Verification items for the finished model (mm, model axes). A direction names the side the tool comes from. Round coordinates to 2 decimals unless told otherwise and drop trailing zeros. Write each loop counter-clockwise with the first axis right and the second up, starting at its lowest first coordinate (ties: lowest second). Pieces come first, ordered by that corner, then holes. Notation, with made-up numbers: M -2,9.5 L 43,9.5 A21 ccw 43,13.5 Z; hole C 52.25,4 d10. An arc over 180 degrees is marked long. Write each question's results on one line, items separated by ' | '.
from build123d import *
from build123d.topology import SkipClean

# Parameters (mm, degrees)
SKETCH1_W                = 50
SKETCH1_H                = 25
SKETCH1_R                = 1.3
SKETCH1_R_2              = 4.5
BOSS_EXTRUDE1_DEPTH      = 2.5
SKETCH2_W                = 50
SKETCH2_H                = 12
BOSS_EXTRUDE2_DEPTH      = 3
SKETCH3_W                = 50
SKETCH3_H                = 28
BOSS_EXTRUDE3_DEPTH      = 3
SKETCH4_R                = 1.3
CUT_EXTRUDE1_DEPTH       = 34.018933962
SKETCH5_W                = 53
SKETCH5_H                = 32.5
SKETCH5_R                = 1.6
SKETCH5_W_2              = 42
SKETCH5_H_2              = 21.5
BOSS_EXTRUDE4_DEPTH      = 4
SKETCH7_R                = 8
CUT_EXTRUDE2_DEPTH       = 5
SKETCH8_W                = 24.55
SKETCH8_H                = 21.5
CUT_EXTRUDE3_DEPTH       = 3.8
BOSS_EXTRUDE6_DEPTH      = 22.95
BOSS_EXTRUDE7_DEPTH      = 2
CUT_EXTRUDE4_START       = -1.2
SKETCH11_R               = 1.6
CUT_EXTRUDE4_DEPTH       = 1.2
SKETCH12_W               = 7
SKETCH12_H               = 21
SKETCH12_R               = 1.6
BOSS_EXTRUDE8_DEPTH      = 7.8
CUT_EXTRUDE5_DEPTH       = 55.054972019
CUT_EXTRUDE5_DEPTH_BACK  = 55.054972019
SKETCH13_W               = 0.7
SKETCH13_H               = 5
SKETCH13_H_2             = 4
CUT_EXTRUDE6_DEPTH       = 78.713850117
CUT_EXTRUDE6_DEPTH_BACK  = 78.713850117
SKETCH14_W               = 28
SKETCH14_H               = 10
SKETCH16_R               = 3
CUT_EXTRUDE8_DEPTH       = 3
SKETCH15_R               = 1.6
CUT_EXTRUDE9_DEPTH       = 5
SKETCH17_W               = 16.3
SKETCH17_H               = 5
CUT_EXTRUDE10_DEPTH      = 3.2
SKETCH18_R               = 1.45
CUT_EXTRUDE11_DEPTH      = 5
CUT_EXTRUDE12_DEPTH      = 54.307527611
CUT_EXTRUDE12_DEPTH_BACK = 54.307527611
SKETCH19_R               = 1.6
CUT_EXTRUDE14_DEPTH      = 60.569224437
CUT_EXTRUDE14_DEPTH_BACK = 60.569224437
SKETCH20_W               = 17.95
SKETCH20_H               = 5
BOSS_EXTRUDE11_START     = 2
SKETCH21_W               = 16.3
SKETCH21_H               = 5
SKETCH21_R               = 1.45
BOSS_EXTRUDE11_DEPTH     = 2


with BuildPart() as part:
    # Sketch1 → Boss-Extrude1 (new, symmetric)
    with BuildSketch(Plane(origin=(0, 0, 0), x_dir=(1, 0, 0), z_dir=(0, 1, 0))):
        Rectangle(SKETCH1_W, SKETCH1_H)
        with Locations(Location((-11.25, 0, 0), (0, 0, 270))):
            Circle(SKETCH1_R, mode=Mode.SUBTRACT)
        with Locations(Location((11.25, 0, 0), (0, 0, 270))):
            Circle(SKETCH1_R_2, mode=Mode.SUBTRACT)
    extrude(amount=BOSS_EXTRUDE1_DEPTH, both=True)

    # Sketch2 → Boss-Extrude2 (add)
    with BuildSketch(Plane.XY.offset(12.5)):
        with Locations((0, 3.5)):
            Rectangle(SKETCH2_W, SKETCH2_H)
    extrude(amount=BOSS_EXTRUDE2_DEPTH)

    # Sketch3 → Boss-Extrude3 (add)
    with BuildSketch(Plane(origin=(0, 9.5, 0), x_dir=(1, 0, 0), z_dir=(0, 1, 0))):
        with Locations((0, -1.5)):
            Rectangle(SKETCH3_W, SKETCH3_H)
    extrude(amount=BOSS_EXTRUDE3_DEPTH)

    # Sketch4 → Cut-Extrude1 (cut, through all)
    with BuildSketch(Plane(origin=(0, 12.5, 0), x_dir=(1, 0, 0), z_dir=(0, 1, 0))):
        with Locations(Location((11.25, 0, 0), (0, 0, 270))):
            Circle(SKETCH4_R)
        with Locations(Location((-11.25, 0, 0), (0, 0, 270))):
            Circle(SKETCH4_R)
    extrude(amount=-CUT_EXTRUDE1_DEPTH, mode=Mode.SUBTRACT)

    # Sketch5 → Boss-Extrude4 (add)
    with BuildSketch(Plane.XZ.offset(2.5)):
        with Locations((21.45, -0.05)):
            Rectangle(SKETCH5_W, SKETCH5_H)
        with Locations(Location((45.75, -5, 0), (0, 0, 270))):
            Circle(SKETCH5_R, mode=Mode.SUBTRACT)
        with Locations(Location((45.75, 4.9, 0), (0, 0, 270))):
            Circle(SKETCH5_R, mode=Mode.SUBTRACT)
        with Locations(Location((-2.85, 4.9, 0), (0, 0, 270))):
            Circle(SKETCH5_R, mode=Mode.SUBTRACT)
        with Locations(Location((-2.85, -5, 0), (0, 0, 270))):
            Circle(SKETCH5_R, mode=Mode.SUBTRACT)
        with Locations((21.45, -0.05)):
            Rectangle(SKETCH5_W_2, SKETCH5_H_2, mode=Mode.SUBTRACT)
    extrude(amount=BOSS_EXTRUDE4_DEPTH)

    # Sketch7 → Cut-Extrude2 (cut)
    with BuildSketch(Plane.XZ.offset(2.5)):
        with Locations(Location((11.25, 0, 0), (0, 0, 270))):
            Circle(SKETCH7_R)
    extrude(amount=-CUT_EXTRUDE2_DEPTH, mode=Mode.SUBTRACT)

    # Sketch8 → Cut-Extrude3 (cut)
    with BuildSketch(Plane.XZ.offset(2.5)):
        with Locations((12.725, -0.05)):
            Rectangle(SKETCH8_W, SKETCH8_H)
    extrude(amount=-CUT_EXTRUDE3_DEPTH, mode=Mode.SUBTRACT)

    # Sketch9 → Boss-Extrude6 (add)
    with BuildSketch(Plane(origin=(25, 0, 0), x_dir=(0, 0, -1), z_dir=(1, 0, 0))):
        Polygon((12.5, 2.5), (-16.2, 2.5), (-16.2, -2.5), (-10.7, -2.5), (-10.7, 1.3), (10.8, 1.3), (10.8, -2.5), (12.5, -2.5), align=None)
    extrude(amount=BOSS_EXTRUDE6_DEPTH)

    # Sketch10 → Boss-Extrude7 (add)
    with BuildSketch(Plane(origin=(47.95, 0, 0), x_dir=(0, 0, -1), z_dir=(1, 0, 0))):
        Polygon((16.3, -2.5), (12.5, -2.5), (12.5, 2.5), (-16.2, 2.5), (-16.2, -6.5), (16.3, -6.5), align=None)
    extrude(amount=BOSS_EXTRUDE7_DEPTH)

    # Sketch11 → Cut-Extrude4 (cut)
    with BuildSketch(Plane.XZ.offset(-1.3).offset(CUT_EXTRUDE4_START)):
        with Locations(Location((-2.85, 4.9, 0), (0, 0, 270))):
            Circle(SKETCH11_R)
        with Locations(Location((-2.85, -5, 0), (0, 0, 270))):
            Circle(SKETCH11_R)
        with Locations(Location((45.75, 4.9, 0), (0, 0, 270))):
            Circle(SKETCH11_R)
        with Locations(Location((45.75, -5, 0), (0, 0, 270))):
            Circle(SKETCH11_R)
    extrude(amount=CUT_EXTRUDE4_DEPTH, mode=Mode.SUBTRACT)

    # Sketch12 → Boss-Extrude8 (add)
    with BuildSketch(Plane.XZ.offset(-1.3)):
        with Locations((46.45, 0.2)):
            Rectangle(SKETCH12_W, SKETCH12_H)
        with Locations(Location((45.75, 4.9, 0), (0, 0, 90))):
            Circle(SKETCH12_R, mode=Mode.SUBTRACT)
        with Locations(Location((45.75, -5, 0), (0, 0, 90))):
            Circle(SKETCH12_R, mode=Mode.SUBTRACT)
    extrude(amount=BOSS_EXTRUDE8_DEPTH)

    # Sketch13 → Cut-Extrude5 (cut, two sides: drawn at the far end of the back side and taken through both)
    with BuildSketch(Plane.ZY.offset(-25).offset(-CUT_EXTRUDE5_DEPTH_BACK)):
        with Locations((15.85, 0)):
            Rectangle(SKETCH13_W, SKETCH13_H)
        with Locations((15.85, -4.5)):
            Rectangle(SKETCH13_W, SKETCH13_H_2)
    extrude(amount=CUT_EXTRUDE5_DEPTH + CUT_EXTRUDE5_DEPTH_BACK, mode=Mode.SUBTRACT)

    # Sketch14 → Cut-Extrude6 (cut, two sides: drawn at the far end of the back side and taken through both)
    with BuildSketch(Plane.ZY.offset(25).offset(-CUT_EXTRUDE6_DEPTH_BACK)):
        with Locations((1.5, 7.5)):
            Rectangle(SKETCH14_W, SKETCH14_H)
    extrude(amount=CUT_EXTRUDE6_DEPTH + CUT_EXTRUDE6_DEPTH_BACK, mode=Mode.SUBTRACT)

    # Sketch16 → Cut-Extrude8 (cut)
    with BuildSketch(Plane(origin=(0, 2.5, 0), x_dir=(1, 0, 0), z_dir=(0, 1, 0))):
        with Locations(Location((-2.85, 5, 0), (0, 0, 270))):
            Circle(SKETCH16_R)
        with Locations(Location((-2.85, -4.9, 0), (0, 0, 270))):
            Circle(SKETCH16_R)
        with Locations(Location((45.75, 5, 0), (0, 0, 270))):
            Circle(SKETCH16_R)
        with Locations(Location((45.75, -4.9, 0), (0, 0, 270))):
            Circle(SKETCH16_R)
    extrude(amount=-CUT_EXTRUDE8_DEPTH, mode=Mode.SUBTRACT)

    # Sketch15 → Cut-Extrude9 (cut)
    with SkipClean():  # the faces are left unmerged after this step: merging them gives an invalid solid
        with BuildSketch(Plane(origin=(0, 2.5, 0), x_dir=(1, 0, 0), z_dir=(0, 1, 0))):
            with Locations(Location((-2.85, 5, 0), (0, 0, 270))):
                Circle(SKETCH15_R)
            with Locations(Location((-2.85, -4.9, 0), (0, 0, 270))):
                Circle(SKETCH15_R)
        extrude(amount=-CUT_EXTRUDE9_DEPTH, mode=Mode.SUBTRACT)

    # Sketch17 → Cut-Extrude10 (cut)
    with SkipClean():  # the faces are left unmerged after this step: merging them gives an invalid solid
        with BuildSketch(Plane.XY.offset(15.5)):
            with Locations((8.9, 0)):
                Rectangle(SKETCH17_W, SKETCH17_H)
            with Locations((31, 0)):
                Rectangle(SKETCH17_W, SKETCH17_H)
        extrude(amount=-CUT_EXTRUDE10_DEPTH, mode=Mode.SUBTRACT)

    # Sketch18 → Cut-Extrude11 (cut)
    with SkipClean():  # the faces are left unmerged after this step: merging them gives an invalid solid
        with BuildSketch(Plane.XY.offset(12.3)):
            with Locations((8.95, 0)):
                Circle(SKETCH18_R)
            with Locations((30.95, 0)):
                Circle(SKETCH18_R)
        extrude(amount=-CUT_EXTRUDE11_DEPTH, mode=Mode.SUBTRACT)

    # Sketch19 → Cut-Extrude12 (cut, two sides: drawn at the far end of the back side and taken through both)
    with SkipClean():  # the faces are left unmerged after this step: merging them gives an invalid solid
        with BuildSketch(Plane(origin=(0, 2.5, 0), x_dir=(1, 0, 0), z_dir=(0, 1, 0)).offset(-CUT_EXTRUDE12_DEPTH_BACK)):
            with Locations(Location((33.75, 0, 0), (0, 0, 270))):
                Circle(SKETCH19_R)
        extrude(amount=CUT_EXTRUDE12_DEPTH + CUT_EXTRUDE12_DEPTH_BACK, mode=Mode.SUBTRACT)

    # Sketch20 → Cut-Extrude14 (cut, two sides: drawn at the far end of the back side and taken through both)
    with SkipClean():  # the faces are left unmerged after this step: merging them gives an invalid solid
        with BuildSketch(Plane.XY.offset(15.5).offset(-CUT_EXTRUDE14_DEPTH_BACK)):
            with Locations((-16.025, 0)):
                Rectangle(SKETCH20_W, SKETCH20_H)
        extrude(amount=CUT_EXTRUDE14_DEPTH + CUT_EXTRUDE14_DEPTH_BACK, mode=Mode.SUBTRACT)

    # Sketch21 → Boss-Extrude11 (add)
    # profile 1 of 3: a face of its own
    with SkipClean():  # the faces are left unmerged after this step: merging them gives an invalid solid
        with BuildSketch(Plane.XY.offset(15.5).offset(BOSS_EXTRUDE11_START)):
            with Locations((8.9, 0)):
                Rectangle(SKETCH21_W, SKETCH21_H)
            with Locations((8.95, 0)):
                Circle(SKETCH21_R, mode=Mode.SUBTRACT)
        # profile 2 of 3: a face of its own
        with BuildSketch(Plane.XY.offset(15.5).offset(BOSS_EXTRUDE11_START)):
            Polygon((0.75, -2.5), (0.75, 2.5), (-7.05, 2.5), (-7.05, -2.5), (-5.05, -2.5), (-5.05, -6.5), (49.95, -6.5), (49.95, 2.5), (39.15, 2.5), (39.15, -2.5), (22.85, -2.5), (22.85, 2.5), (17.05, 2.5), (17.05, -2.5), align=None)
        # profile 3 of 3: a face of its own
        with BuildSketch(Plane.XY.offset(15.5).offset(BOSS_EXTRUDE11_START)):
            with Locations((31, 0)):
                Rectangle(SKETCH21_W, SKETCH21_H)
            with Locations((30.95, 0)):
                Circle(SKETCH21_R, mode=Mode.SUBTRACT)
        extrude(amount=-BOSS_EXTRUDE11_DEPTH)


solid = part.part
1) Sectioned sample at D-D, the plane z = -5. Count the separate pieces of the cut face and the enclosed holes in it, and give its area (3 significant figures).
Calculated:
separate pieces: 5 | enclosed holes: 0 | area: 86.5 mm²
2) Sectioned sample at B-B, the plane x = 11.25. Record the cut outline in (y, z).
Calculated:
outline: M -6.5,-16.3 L -2.5,-16.3 L -2.5,-12.5 L 2.5,-12.5 L 2.5,-8 L 1.3,-8 L 1.3,-10.8 L -6.5,-10.8 Z; M -6.5,10.7 L 1.3,10.7 L 1.3,8 L 2.5,8 L 2.5,12.3 L -2.5,12.3 L -2.5,15.5 L 2.5,15.5 L 2.5,17.5 L -6.5,17.5 Z
3) Sectioned sample at A-A, the plane z = 0. Record the cut outline in (x, y).
Calculated:
outline: M -7.05,-2.5 L -5.05,-2.5 L -5.05,-6.5 L 0.45,-6.5 L 0.45,1.3 L 3.25,1.3 L 3.25,2.5 L -7.05,2.5 Z; M 19.25,1.3 L 32.15,1.3 L 32.15,2.5 L 19.25,2.5 Z; M 35.35,1.3 L 42.95,1.3 L 42.95,-2.5 L 42.45,-2.5 L 42.45,-6.5 L 49.95,-6.5 L 49.95,2.5 L 35.35,2.5 Z
4) Draft check along X on faces 5 (the flat face through (0.45, -3, 0)), 6 (the flat face through (21, -2, 17.5)), 7 (the flat face through (-4.1, -0.5, 6.2)), 8 (the flat face through (-5.05, -4, 1)). Enter one of: pulls with the +X half, pulls with the -X half, needs draft (parallel to the pull), parting line crosses it, or undercut.
Calculated:
face 5: undercut | face 6: needs draft | face 7: undercut | face 8: pulls with the -X half
5) Access from +Z, -Z, +X, -X, +Y, -Y to the whole of each face (thin tool, end or side, straight path). Record for faces 1 (the flat face through (22, -2.5, -14)), 2 (the cylindrical face through (29.5, 0.06, 16.51)), 3 (the flat face through (45, -1, -10.3)), 4 (the flat face through (31, 2, 12.3)).
Calculated:
face 1: -Z, +X, -X, +Y | face 2: +Z | face 3: none | face 4: +Y
6) Depth check by flat-ended pin: P1, Ø6, axis at x = 6.5, z = -2, coming from the +Y side; P2, Ø2.5, axis at x = 30.95, y = 0, coming from the +Z side; P3, Ø3, axis at x = -2.85, z = -5, coming from the -Y side (3 decimals); P4, Ø4, axis at x = -2.85, z = 4.9, coming from the +Y side. Enter the tip coordinate at first touch or a pass-through.
Calculated:
P1: stops at y = 2.5 | P2: stops at z = -10.8 | P3: passes through | P4: stops at y = -0.5
7) Material ranges on line 1 (X direction, y = 0.7, z = 4.9); line 2 (X direction, y = -1.4, z = 4.9); line 3 (Z direction, x = 45.75, y = -1), recorded low to high. Write a range as [from, to].
Calculated:
line 1: x = [-7.05, -5.85], [0.15, 0.45], [48.75, 49.95] | line 2: x = [-7.05, -4.45], [-1.25, 0.45], [42.95, 44.15], [47.35, 49.95] | line 3: z = [-12.5, -10.8], [-10.3, -6.6], [-3.4, 3.3], [6.5, 17.5]
8) Sectioned sample at C-C, the plane y = -4.5. Record the cut outline in (x, z), and give its area (3 significant figures).
Calculated:
outline: M -5.05,-16.3 L 49.95,-16.3 L 49.95,17.5 L -5.05,17.5 Z; hole C -2.85,-5 d3.2; hole C -2.85,4.9 d3.2; hole M 0.45,-10.8 L 42.45,-10.8 L 42.45,10.7 L 0.45,10.7 Z; hole C 45.75,-5 d3.2; hole C 45.75,4.9 d3.2 | area: 924 mm²
